The model under review builds one solid part; all positions refer to its coordinate system, in mm. A direction names the side the tool comes from. Round coordinates to 2 decimals unless told otherwise and drop trailing zeros. Loops run counter-clockwise (first coordinate to the right, second up) from the corner with the lowest first, then second, coordinate; pieces in that order, holes last. Notation, with made-up numbers: (42.5, -15) -> (65.5, -15) arc R15 cw to (65.5, -3) -> close; hole circle Ø5 at (41.25, 52). An arc over 180 degrees is marked (long way). Use a Markdown table: item, result. Add a question column.
1) Consider section D-D on y = -23. Give the boundary of the cut face in (x, z), plus the area to 3 significant figures.
2) Consider section B-B on y = 0. Give the boundary of the cut face in (x, z), plus the area to 3 significant figures.
3) Mouldability with a two-part tool opening along X and no side actions: class faces 3 (the flat face through (-1, -40, 22)), 4 (the cylindrical face through (-16, -12, 17)), 5 (the flat face through (22.48, -26.33, 32.17)) as released by +X, released by -X, zero draft, split by the parting line, or undercut.
4) Consider section A-A on x = 0. Give the boundary of the cut face in (y, z).
5) Insertion check: pin 1 (8 mm diameter, centred on y = -20.5, z = 30, fed in from +X) (3 decimals). The pin has a flat end and moves straight along its axis. Give the tip position at first contact, or say it passes through.
6) For faces 1 (the flat face through (-8.5, 30, 32.2)), 2 (the flat face through (-12, 40, 17)), list the 3-axis set-ups (+Z, -Z, +X, -X, +Y, -Y) from which the entire face can be reached by the end or side of a thin tool; tool diameter is ignored.
7) Wall thickness on probe 1 along X at (y, z) = (0, 16.5); probe 2 along Y at (x, z) = (0, 13); probe 3 along Z at (x, y) = (40, -8.5): over which ranges is each line inside the solid? List them lowest first.
8) Consider section C-C on z = 17.5. Give the boundary of the cut face in (x, y), plus the area to 3 significant figures.
from build123d import *

# Parameters (mm, degrees)
F0_W     = 100
F0_H     = 80
F1_DEPTH = 44
F2_R     = 20
F3_DEPTH = 44.001
F5_DEPTH = 24


with BuildPart() as f1:
    # F0 (on Top) → F1 (new body)
    with BuildSketch(Plane.XY):
        Rectangle(F0_W, F0_H)
    extrude(amount=F1_DEPTH)

    # F2 (on face) → F3 (cut, through all)
    with BuildSketch(Plane.XY.offset(44)):
        Circle(F2_R)
    extrude(amount=-F3_DEPTH, mode=Mode.SUBTRACT)

    # F4 (on face) → F5 (cut)
    with BuildSketch(Plane.XY.offset(44)):
        Polygon((50, 40), (-14, 40), (30, -40), (50, -40), align=None)
    extrude(amount=-F5_DEPTH, mode=Mode.SUBTRACT)


solid = f1.part
Result set:
| question | item | result |
|---|---|---|
| 1 | outline | (-50, 0) -> (50, 0) -> (50, 20) -> (20.65, 20) -> (20.65, 44) -> (-50, 44) -> close |
| 1 | area | 3,700 mm2 |
| 2 | outline | (-50, 0) -> (-20, 0) -> (-20, 44) -> (-50, 44) -> close; (20, 0) -> (50, 0) -> (50, 20) -> (20, 20) -> close |
| 2 | area | 1,920 mm2 |
| 3 | face 3 | zero draft |
| 3 | face 4 | undercut |
| 3 | face 5 | released by +X |
| 4 | outline | (-40, 0) -> (-20, 0) -> (-20, 44) -> (-40, 44) -> close; (20, 0) -> (40, 0) -> (40, 20) -> (20, 20) -> close |
| 5 | pin 1 | x = 21.475 |
| 6 | face 1 | +Z, +X, +Y |
| 6 | face 2 | +Z, -Z, +X, -X, +Y |
| 7 | probe 1 | -50 to -20, 20 to 50 |
| 7 | probe 2 | -40 to -20, 20 to 40 |
| 7 | probe 3 | 0 to 20 |
| 8 | outline | (-50, -40) -> (50, -40) -> (50, 40) -> (-50, 40) -> close; hole circle Ø40 at (0, 0) |
| 8 | area | 6,740 mm2 |
